CAD build for the part. Positions are in the model's coordinates, mm. A direction names the side the tool comes from. Round coordinates to 2 decimals unless told otherwise and drop trailing zeros. Order: outer loops, then holes, each group sorted by start corner. A loop starts at its lowest first (then second) coordinate and runs counter-clockwise, first axis right, second up. Notation, with made-up numbers: M 57.5,-4.75 L 64.5,-4.75 A30 ccw 64.5,27.25 Z; hole C -0.75,-39 d1. An arc over 180 degrees is marked long. Answer as a JSON object with one key per item and string values. Group by question number.
```python
from build123d import *

# Parameters (mm, degrees)
SKETCH_1_R          = 9
SKETCH_1_R_2        = 12
SKETCH_1_R_3        = 1.5
EXTRUDE_1_DEPTH     = 3
SKETCH_3_R          = 1.5
CUT_EXTRUDE_1_DEPTH = 3
SKETCH_4_R          = 11
SKETCH_4_R_2        = 9
CUT_EXTRUDE_2_DEPTH = 1.5


with BuildPart() as part:
    # Sketch 1 → Extrude 1 (new body)
    with BuildSketch(Plane(origin=(0, 0, 0), x_dir=(1, 0, 0), z_dir=(0, 1, 0))):
        with BuildLine():
            Line((-69.123560149, -19.49646317), (13.276439851, -58.69646317))
            ThreePointArc((13.276439851, -58.69646317), (26.88689597, -63.404534956), (41.2, -65))
            ThreePointArc((41.2, -65), (104.604534956, -14.31310403), (69.123560149, 58.69646317))
            Line((69.123560149, 58.69646317), (-13.276439851, 97.89646317))
            ThreePointArc((-13.276439851, 97.89646317), (-99.89646317, 67.123560149), (-69.123560149, -19.49646317))
        make_face()
        with Locations(Location((41.2, 0, 0), (0, 0, 270))):
            Circle(SKETCH_1_R, mode=Mode.SUBTRACT)
        with Locations(Location((-41.2, 39.2, 0), (0, 0, 270))):
            Circle(SKETCH_1_R_2, mode=Mode.SUBTRACT)
        with Locations(Location((87.2, 0, 0), (0, 0, 270))):
            Circle(SKETCH_1_R_3, mode=Mode.SUBTRACT)
        with Locations(Location((55.414781741, -43.74859975, 0), (0, 0, 270))):
            Circle(SKETCH_1_R_3, mode=Mode.SUBTRACT)
        with Locations(Location((3.985218259, -27.038121605, 0), (0, 0, 270))):
            Circle(SKETCH_1_R_3, mode=Mode.SUBTRACT)
        with Locations(Location((3.985218259, 27.038121605, 0), (0, 0, 270))):
            Circle(SKETCH_1_R_3, mode=Mode.SUBTRACT)
        with Locations(Location((55.414781741, 43.74859975, 0), (0, 0, 270))):
            Circle(SKETCH_1_R_3, mode=Mode.SUBTRACT)
        with Locations(Location((61.2, 0, 0), (0, 0, 270))):
            Circle(SKETCH_1_R_3, mode=Mode.SUBTRACT)
        with Locations(Location((31.2, -17.320508076, 0), (0, 0, 270))):
            Circle(SKETCH_1_R_3, mode=Mode.SUBTRACT)
        with Locations(Location((31.2, 17.320508076, 0), (0, 0, 270))):
            Circle(SKETCH_1_R_3, mode=Mode.SUBTRACT)
        with Locations(Location((36.7, -36.5, 0), (0, 0, 270))):
            Circle(SKETCH_1_R_3, mode=Mode.SUBTRACT)
        with Locations(Location((36.7, 36.5, 0), (0, 0, 270))):
            Circle(SKETCH_1_R_3, mode=Mode.SUBTRACT)
        with Locations(Location((-83.95, 0, 0), (0, 0, 270))):
            Circle(SKETCH_1_R_3, mode=Mode.SUBTRACT)
        with Locations(Location((-41.2, 97.201745663, 0), (0, 0, 270))):
            Circle(SKETCH_1_R_3, mode=Mode.SUBTRACT)
        with Locations(Location((16.801745663, 39.2, 0), (0, 0, 270))):
            Circle(SKETCH_1_R_3, mode=Mode.SUBTRACT)
        with Locations(Location((-41.2, -18.801745663, 0), (0, 0, 270))):
            Circle(SKETCH_1_R_3, mode=Mode.SUBTRACT)
        with Locations(Location((-83.95, 80, 0), (0, 0, 270))):
            Circle(SKETCH_1_R_3, mode=Mode.SUBTRACT)
        with Locations(Location((6.05, 80, 0), (0, 0, 270))):
            Circle(SKETCH_1_R_3, mode=Mode.SUBTRACT)
        with Locations(Location((6.05, 18, 0), (0, 0, 270))):
            Circle(SKETCH_1_R_3, mode=Mode.SUBTRACT)
        with Locations(Location((6.05, -18, 0), (0, 0, 270))):
            Circle(SKETCH_1_R_3, mode=Mode.SUBTRACT)
        with Locations(Location((-103.2, 39.2, 0), (0, 0, 270))):
            Circle(SKETCH_1_R_3, mode=Mode.SUBTRACT)
    extrude(amount=EXTRUDE_1_DEPTH)

    # Sketch 3 → Cut-Extrude 1 (cut)
    with BuildSketch(Plane(origin=(0, 3, 0), x_dir=(1, 0, 0), z_dir=(0, 1, 0))):
        with Locations(Location((-10.807832752, -39.489084979, 0), (0, 0, 270))):
            Circle(SKETCH_3_R)
        with Locations(Location((45.80954965, -57.818289079, 0), (0, 0, 270))):
            Circle(SKETCH_3_R)
        with Locations(Location((93.576881971, -24.917157442, 0), (0, 0, 270))):
            Circle(SKETCH_3_R)
        with Locations(Location((88.967332321, 32.901131637, 0), (0, 0, 270))):
            Circle(SKETCH_3_R)
        with Locations(Location((39.026482133, 65.264678963, 0), (0, 0, 270))):
            Circle(SKETCH_3_R)
    extrude(amount=-CUT_EXTRUDE_1_DEPTH, mode=Mode.SUBTRACT)

    # Sketch 4 → Cut-Extrude 2 (cut)
    with BuildSketch(Plane.XZ):
        with Locations((41.2, 0)):
            Circle(SKETCH_4_R)
        with Locations((41.2, 0)):
            Circle(SKETCH_4_R_2, mode=Mode.SUBTRACT)
    extrude(amount=-CUT_EXTRUDE_2_DEPTH, mode=Mode.SUBTRACT)


solid = part.part
```
Item 1: Two-plate mould, pull along X, no slides. Class faces 3 (the face through (-1, 3, -21)), 4 (the face through (-28.5, 1.479, 38.822)), 5 (the face through (32, 1.5, 0)): +X half, -X half, draft (parallel to the pull), parting line (faces both ways), or undercut.
Item 2: Cut at B-B, the plane y = 2.15. Give the number of separate pieces and of enclosed holes in the cut face, and give its area (3 significant figures).
Item 3: Flat gauge pins, fed straight in: pin 1 Ø1.5 at (y, z) = (1.5, -38) entering from -X; pin 2 Ø2.5 at (x, z) = (3.99, -27.04) entering from +Y. Where does each tip first touch, or does it go through?
Item 4: Cut at A-A, the plane x = -45.5. Give the cut face in (y, z), and give its area (3 significant figures).
Item 5: 3-axis set-ups, long thin cutter, end or side, ignore diameter. For faces 1 (the face through (28.5, 1.479, -78.022)), 2 (the face through (51.361, 0.74, -4.213)): which of +Z, -Z, +X, -X, +Y, -Y reach the whole face in a straight line?
Item 6: Drill centre lines: line 1 (X direction, y = 0.35, z = -39.5); line 2 (X direction, y = 2.4, z = 0); line 3 (X direction, y = 0.7, z = -39.2). Where is each one in solid material? Low to high. Write a range as [from, to].
Item 7: Cut at C-C, the plane x = -16. Give the cut face in (y, z).
Response values:
{
 "1": {"face 3": "draft", "face 4": "-X half", "face 5": "undercut"},
 "2": {"separate pieces": "1", "enclosed holes": "26", "area": "24,300 mm^2"},
 "3": {"pin 1": "x = -106.2", "pin 2": "through"},
 "4": {"outline": "M 0,-104.06 L 3,-104.06 L 3,-50.4 L 0,-50.4 Z; M 0,-28 L 3,-28 L 3,30.73 L 0,30.73 Z", "area": "337 mm^2"},
 "5": {"face 1": "-Z, +X, +Y, -Y", "face 2": "-Y"},
 "6": {"line 1": "[-106.2, -104.67], [-101.73, -53.2], [-29.2, 15.33], [18.27, 92.82]", "line 2": "[-93.05, -85.45], [-82.45, 32.2], [50.2, 59.7], [62.7, 85.7], [88.7, 106.2]", "line 3": "[-106.2, -104.7], [-101.7, -53.2], [-29.2, 15.3], [18.3, 93.05]"},
 "7": {"outline": "M 0,-99.12 L 3,-99.12 L 3,44.77 L 0,44.77 Z"}
}
